The model under review builds one solid part; all positions refer to its coordinate system, in mm. Coordinates: 2 decimals unless noted, no trailing zeros. Loops run counter-clockwise (first coordinate to the right, second up) from the corner with the lowest first, then second, coordinate; pieces in that order, holes last. Notation, with made-up numbers: M 67.25,88 L 105.25,88 A21 cw 105.25,120 Z; hole C 58,-31 d4. An arc over 180 degrees is marked long. One line per item, written item: value.
```python
from build123d import *

# Parameters (mm, degrees)
CYLINDER003_R          = 1.6
CYLINDER003_DEPTH      = 10
FUSION_PLACEMENT_ANGLE = 90
BOX002_W               = 12
BOX002_H               = 10
BOX002_DEPTH           = 6
BOX001_W               = 12
BOX001_H               = 10
BOX001_DEPTH           = 6
CYLINDER002_R          = 3
CYLINDER002_DEPTH      = 10
CYLINDER001_R          = 5
CYLINDER001_DEPTH      = 10
CYLINDER_R             = 3
CYLINDER_DEPTH         = 10
BOX_W                  = 66
BOX_H                  = 2
BOX_DEPTH              = 49


with BuildPart() as zylinder003:
    # Cylinder003 → Cylinder003 (new body)
    with BuildSketch(Plane.XY.offset(-6)):
        Circle(CYLINDER003_R)
    extrude(amount=CYLINDER003_DEPTH)


with BuildPart() as fusion:
    # Cone003 → Cone003 (revolve)
    with BuildSketch(Plane.XZ):
        Polygon((0, 0), (4, 4), (0, 4), align=None)
    revolve(axis=Axis((0, 0, 0), (0, 0, 1)))

    # Fusion: union Zylinder003
    add(zylinder003.part)


with BuildPart() as fusion_1:
    # Fusion placement: moved
    add(fusion.part.moved(Location((-2.4, 34, 9))).rotate(Axis((-2.4, 34, 9), (0, 1, 0)), FUSION_PLACEMENT_ANGLE))


with BuildPart() as obj1:
    # Box002 → Box002 (new body)
    with BuildSketch(Plane(origin=(4, 67.5, -1.5), x_dir=(0, -1, 0), z_dir=(0, 0, -1))):
        with Locations((6, 5)):
            Rectangle(BOX002_W, BOX002_H)
    extrude(amount=BOX002_DEPTH)


with BuildPart() as obj2:
    # Box001 → Box001 (new body)
    with BuildSketch(Plane(origin=(3, 10.5, -1.5), x_dir=(0, -1, 0), z_dir=(0, 0, -1))):
        with Locations((6, 5)):
            Rectangle(BOX001_W, BOX001_H)
    extrude(amount=BOX001_DEPTH)


with BuildPart() as zylinder002:
    # Cylinder002 → Cylinder002 (new body)
    with BuildSketch(Plane(origin=(-5.5, 55.5, -4.5), x_dir=(0, 0, -1), z_dir=(1, 0, 0))):
        Circle(CYLINDER002_R)
    extrude(amount=CYLINDER002_DEPTH)


with BuildPart() as zylinder001:
    # Cylinder001 → Cylinder001 (new body)
    with BuildSketch(Plane(origin=(-5, 40.5, -15.9), x_dir=(0, 0, -1), z_dir=(1, 0, 0))):
        Circle(CYLINDER001_R)
    extrude(amount=CYLINDER001_DEPTH)


with BuildPart() as zylinder:
    # Cylinder → Cylinder (new body)
    with BuildSketch(Plane(origin=(-5.5, 10.5, -4.5), x_dir=(0, 0, -1), z_dir=(1, 0, 0))):
        Circle(CYLINDER_R)
    extrude(amount=CYLINDER_DEPTH)


with BuildPart() as cut005:
    # Box → Box (new body)
    with BuildSketch(Plane(origin=(0, 66, 20), x_dir=(0, -1, 0), z_dir=(0, 0, -1))):
        with Locations((33, 1)):
            Rectangle(BOX_W, BOX_H)
    extrude(amount=BOX_DEPTH)

    # Cut: cut Zylinder
    add(zylinder.part, mode=Mode.SUBTRACT)

    # Cut001: cut Zylinder001
    add(zylinder001.part, mode=Mode.SUBTRACT)

    # Cut002: cut Zylinder002
    add(zylinder002.part, mode=Mode.SUBTRACT)

    # Cut003: cut obj2
    add(obj2.part, mode=Mode.SUBTRACT)

    # Cut004: cut obj1
    add(obj1.part, mode=Mode.SUBTRACT)

    # Cut005: cut Fusion
    add(fusion_1.part, mode=Mode.SUBTRACT)


solid = cut005.part
```
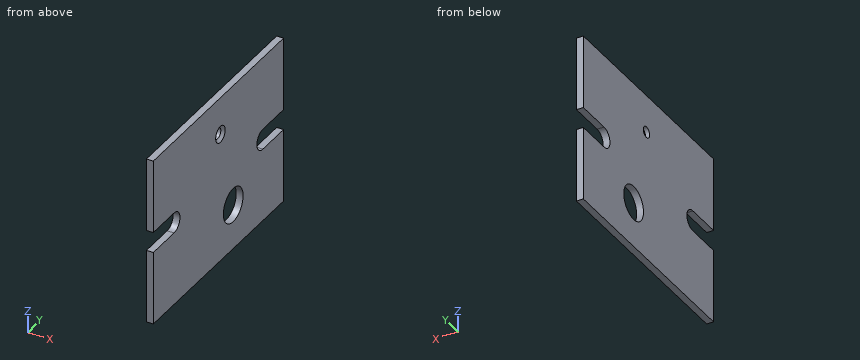
(1) To check wall thickness, follow L1, parallel to Y at x = -1.3, z = -15.9; L2, parallel to Z at x = -0.45, y = 6; L3, parallel to Z at x = -0.95, y = 40.5. State the ranges of each line that lie inside material, in increasing order. Write a range as [from, to].
Checks:
L1: [0, 35.5], [45.5, 66]
L2: [-29, -7.5], [-1.5, 20]
L3: [-29, -20.9], [-10.9, 20]
(2) Add section A-A on z = -15.9. State the section outline as (x, y) points.
Checks:
outline: M -2,0 L 0,0 L 0,35.5 L -2,35.5 Z; M -2,45.5 L 0,45.5 L 0,66 L -2,66 Z
(3) Insertion check: pin 1 Ø11.5 at (y, z) = (40.5, -15.9) entering from -X. The pin has a flat end and moves straight along its axis. Give the tip position at first contact, or say it passes through.
Checks:
pin 1: x = -2
(4) Add section C-C on x = -0.4. State the section outline as (y, z) points, then the cut area to 3 significant figures.
Checks:
outline: M 0,-29 L 66,-29 L 66,-7.5 L 55.5,-7.5 A3 cw 55.5,-1.5 L 66,-1.5 L 66,20 L 0,20 L 0,-1.5 L 10.5,-1.5 A3 cw 10.5,-7.5 L 0,-7.5 Z; hole C 34,9 d4; hole C 40.5,-15.9 d10
area: 2,990 mm^2
(5) Add section D-D on z = -4.5. State the section outline as (x, y) points.
Checks:
outline: M -2,13.5 L 0,13.5 L 0,52.5 L -2,52.5 Z
(6) Add section B-B on y = 40.5. State the section outline as (x, z) points.
Checks:
outline: M -2,-29 L 0,-29 L 0,-20.9 L -2,-20.9 Z; M -2,-10.9 L 0,-10.9 L 0,20 L -2,20 Z
